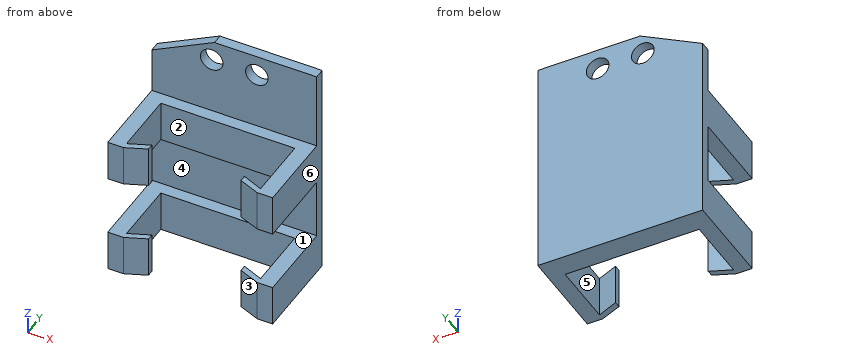
```python
from build123d import *

# Parameters (mm, degrees)
SKETCH3_R           = 2.7813
BOSS_EXTRUDE3_DEPTH = 2.54
SKETCH4_W           = 3.81
SKETCH4_H           = 40.386
BOSS_EXTRUDE4_DEPTH = 20.32
SKETCH5_W           = 40.386
SKETCH5_H           = 1.524
BOSS_EXTRUDE5_DEPTH = 5.08
SKETCH6_W           = 40.386
SKETCH6_H           = 1.524
BOSS_EXTRUDE6_DEPTH = 5.08
SKETCH7_W           = 40.64
SKETCH7_H           = 20.32
CUT_EXTRUDE1_DEPTH  = 5.08
SKETCH11_W          = 40.64
SKETCH11_H          = 35.306
BOSS_EXTRUDE7_DEPTH = 2.9718
BOSS_EXTRUDE8_DEPTH = 35.306
SKETCH8_W           = 14.986
SKETCH8_H           = 20.32
CUT_EXTRUDE2_DEPTH  = 41.64
CUT_EXTRUDE3_DEPTH  = 36.306
SKETCH14_R          = 3.81
SKETCH14_R_2        = 2.7813
BOSS_EXTRUDE9_DEPTH = 2.54
CUT_EXTRUDE4_DEPTH  = 23.86


with BuildPart() as part:
    # Sketch3 → Boss-Extrude3 (new body)
    with BuildSketch(Plane(origin=(0, 0, 0), x_dir=(1, 0, 0), z_dir=(0, 1, 0))):
        Polygon((-11.517251908, 12.440983784), (29.122748092, 12.440983784), (29.122748092, -34.564151764), (29.122748092, -42.169016216), (18.885256114, -42.169016216), (-11.517251908, -42.169016216), align=None)
        with Locations((3.240148092, -37.089016216)):
            Circle(SKETCH3_R, mode=Mode.SUBTRACT)
        with Locations((14.365348092, -37.089016216)):
            Circle(SKETCH3_R, mode=Mode.SUBTRACT)
    extrude(amount=BOSS_EXTRUDE3_DEPTH)

    # Sketch4 → Boss-Extrude4 (add)
    with BuildSketch(Plane.XZ):
        with Locations((-9.612251908, 7.752016216)):
            Rectangle(SKETCH4_W, SKETCH4_H)
        with Locations((27.217748092, 7.752016216)):
            Rectangle(SKETCH4_W, SKETCH4_H)
    extrude(amount=BOSS_EXTRUDE4_DEPTH)

    # Sketch5 → Boss-Extrude5 (add)
    with BuildSketch(Plane(origin=(-7.707251908, 0, 0), x_dir=(0, 0, -1), z_dir=(1, 0, 0))):
        with Locations((-7.752016216, -19.558)):
            Rectangle(SKETCH5_W, SKETCH5_H)
    extrude(amount=BOSS_EXTRUDE5_DEPTH)

    # Sketch6 → Boss-Extrude6 (add)
    with BuildSketch(Plane.ZY.offset(-25.312748092)):
        with Locations((7.752016216, -19.558)):
            Rectangle(SKETCH6_W, SKETCH6_H)
    extrude(amount=BOSS_EXTRUDE6_DEPTH)

    # Sketch7 → Cut-Extrude1 (cut)
    with BuildSketch(Plane.XY.offset(27.945016216)):
        with Locations((8.802748092, -10.16)):
            Rectangle(SKETCH7_W, SKETCH7_H)
    extrude(amount=-CUT_EXTRUDE1_DEPTH, mode=Mode.SUBTRACT)

    # Sketch11 → Boss-Extrude7 (add)
    with BuildSketch(Plane.XZ):
        with Locations((8.802748092, 5.212016216)):
            Rectangle(SKETCH11_W, SKETCH11_H)
    extrude(amount=BOSS_EXTRUDE7_DEPTH)

    # Sketch12 → Boss-Extrude8 (add)
    with BuildSketch(Plane.XY.offset(22.865016216)):
        Polygon((-7.707251908, -18.796), (-2.593407451, -16.66881978), (-2.627251908, -18.796), align=None)
        Polygon((20.232748092, -18.796), (20.232748092, -16.66881978), (25.312748092, -18.796), align=None)
    extrude(amount=-BOSS_EXTRUDE8_DEPTH)

    # Sketch8 → Cut-Extrude2 (cut, through all)
    with BuildSketch(Plane(origin=(29.122748092, 0, 0), x_dir=(0, 0, -1), z_dir=(1, 0, 0))):
        with Locations((-5.212016216, -10.16)):
            Rectangle(SKETCH8_W, SKETCH8_H)
    extrude(amount=-CUT_EXTRUDE2_DEPTH, mode=Mode.SUBTRACT)

    # Sketch13 → Cut-Extrude3 (cut, through all)
    with BuildSketch(Plane.XY.offset(22.865016216)):
        Polygon((-2.618031664, -18.216492377), (-7.660745747, -20.32), (-2.627251908, -20.32), (-2.627251908, -18.796), align=None)
        Polygon((20.232748092, -18.294602636), (20.232748092, -20.32), (25.312748092, -20.32), align=None)
    extrude(amount=-CUT_EXTRUDE3_DEPTH, mode=Mode.SUBTRACT)

    # Sketch14 → Boss-Extrude9 (add)
    with BuildSketch(Plane.XZ):
        with Locations((3.240148092, 37.089016216)):
            Circle(SKETCH14_R)
        with Locations((3.240148092, 37.089016216)):
            Circle(SKETCH14_R_2, mode=Mode.SUBTRACT)
        with Locations((14.365348092, 37.089016216)):
            Circle(SKETCH14_R)
        with Locations((14.365348092, 37.089016216)):
            Circle(SKETCH14_R_2, mode=Mode.SUBTRACT)
    extrude(amount=-BOSS_EXTRUDE9_DEPTH)

    # Sketch15 → Cut-Extrude4 (cut, through all)
    with BuildSketch(Plane(origin=(0, 2.54, 0), x_dir=(1, 0, 0), z_dir=(0, 1, 0))):
        Polygon((-11.517251908, -42.169016216), (3.92724007, -42.169016216), (-11.517251908, -34.183083779), align=None)
    extrude(amount=-CUT_EXTRUDE4_DEPTH, mode=Mode.SUBTRACT)


solid = part.part
```
Geometry check sheet. Reference: the model listing, model coordinates, mm. Face numbers are marked on the shaded views. A direction names the side the tool comes from. Coordinates: 2 decimals unless noted, no trailing zeros. Write each loop counter-clockwise with the first axis right and the second up, starting at its lowest first coordinate (ties: lowest second). Pieces come first, ordered by that corner, then holes. Notation, with made-up numbers: M 45.25,59.5 L 89.25,59.5 A23 ccw 89.25,74.5 Z; hole C 35,26.5 d8. An arc over 180 degrees is marked long. Answer as a JSON object with one key per item and string values.
1. Section check C-C, the plane z = 15. Enter the section's corners in (x, y), plus the area to 3 significant figures.
Answers below:
{"outline": "M -11.52,-20.32 L -7.66,-20.32 L -2.62,-18.22 L -2.59,-16.67 L -7.71,-18.8 L -7.71,-2.97 L 25.31,-2.97 L 25.31,-18.8 L 20.23,-16.67 L 20.23,-18.29 L 25.31,-20.32 L 29.12,-20.32 L 29.12,2.54 L -11.52,2.54 Z", "area": "372 mm²"}
2. Draft check along X on the marked faces 4, 5 and 6. Enter one of: released by +X, released by -X, zero draft, split by the parting line, or undercut.
Answers below:
{"face 4": "zero draft", "face 5": "undercut", "face 6": "released by +X"}
3. Tool access check on the marked faces 1, 2 and 3. Record the directions out of +Z, -Z, +X, -X, +Y, -Y that give a thin tool (end or side, any length) a straight path to the whole face; none if there is none.
Answers below:
{"face 1": "+X, -X, -Y", "face 2": "+Z, -Z", "face 3": "+Z, -Z, -Y"}
4. Section check D-D, the plane y = -12.75. Enter the section's corners in (x, z).
Answers below:
{"outline": "M -11.52,-12.44 L -7.71,-12.44 L -7.71,-2.28 L -11.52,-2.28 Z; M -11.52,12.71 L -7.71,12.71 L -7.71,22.87 L -11.52,22.87 Z; M 25.31,-12.44 L 29.12,-12.44 L 29.12,-2.28 L 25.31,-2.28 Z; M 25.31,12.71 L 29.12,12.71 L 29.12,22.87 L 25.31,22.87 Z"}
5. Scan lines: L1, parallel to Z at x = 26.5, y = -17.5; L2, parallel to X at y = -6.5, z = -2.5; L3, parallel to Y at x = 16.5, z = -3.5. Record each from-to range of solid material in increasing order.
Answers below:
{"L1": "z = -12.44 to -2.28, 12.71 to 22.87", "L2": "x = -11.52 to -7.71, 25.31 to 29.12", "L3": "y = -2.97 to 2.54"}
6. Section check A-A, the plane x = 8. Enter the section's corners in (y, z), plus the area to 3 significant figures.
Answers below:
{"outline": "M -2.97,-12.44 L 2.54,-12.44 L 2.54,42.17 L 0,42.17 L 0,22.87 L -2.97,22.87 L -2.97,12.71 L 0,12.71 L 0,-2.28 L -2.97,-2.28 Z", "area": "199 mm²"}
7. Section check B-B, the plane y = -1. Enter the section's corners in (x, z).
Answers below:
{"outline": "M -11.52,-12.44 L 29.12,-12.44 L 29.12,-2.28 L -11.52,-2.28 Z; M -11.52,12.71 L 29.12,12.71 L 29.12,22.87 L -11.52,22.87 Z"}
8. Go/stop test with flat-tipped pins: pin 1 Ø4 at (x, y) = (24, -12) entering from +Z (3 decimals); pin 2 Ø8 at (x, z) = (16, -6.5) entering from -Y; pin 3 Ø4.5 at (x, z) = (14.5, 9) entering from -Y. Record where each tip stops, or that it passes through.
Answers below:
{"pin 1": "stops at z = 22.865", "pin 2": "stops at y = -2.97", "pin 3": "stops at y = 0"}
